from build123d import *

# Parameters (mm, degrees)
SKETCH1_R           = 1.65
BOSS_EXTRUDE1_DEPTH = 16
CUT_EXTRUDE1_START  = -9
CUT_EXTRUDE1_DEPTH  = 9
CUT_EXTRUDE2_DEPTH  = 4
SKETCH4_R           = 1.65
CUT_EXTRUDE3_DEPTH  = 7
CUT_EXTRUDE4_DEPTH  = 4


with BuildPart() as part:
    # Sketch1 → Boss-Extrude1 (new body)
    with BuildSketch(Plane.XY):
        with BuildLine():
            Line((36.52, 7), (33.22, 7))
            ThreePointArc((33.22, 7), (32.866446609, 7.146446609), (32.72, 7.5))
            Line((32.72, 7.5), (32.72, 15.5))
            ThreePointArc((32.72, 15.5), (32.573553391, 15.853553391), (32.22, 16))
            Line((32.22, 16), (4.8, 16))
            ThreePointArc((4.8, 16), (4.446446609, 15.853553391), (4.3, 15.5))
            Line((4.3, 15.5), (4.3, 7.5))
            ThreePointArc((4.3, 7.5), (4.153553391, 7.146446609), (3.8, 7))
            Line((3.8, 7), (0.5, 7))
            ThreePointArc((0.5, 7), (0.146446609, 6.853553391), (0, 6.5))
            Line((0, 6.5), (0, 0.5))
            ThreePointArc((0, 0.5), (0.146446609, 0.146446609), (0.5, 0))
            Line((0.5, 0), (36.52, 0))
            ThreePointArc((36.52, 0), (36.873553391, 0.146446609), (37.02, 0.5))
            Line((37.02, 0.5), (37.02, 6.5))
            ThreePointArc((37.02, 6.5), (36.873553391, 6.853553391), (36.52, 7))
        make_face()
        with Locations((8.81, 11.5)):
            Circle(SKETCH1_R, mode=Mode.SUBTRACT)
        with Locations((28.21, 11.5)):
            Circle(SKETCH1_R, mode=Mode.SUBTRACT)
    extrude(amount=BOSS_EXTRUDE1_DEPTH)

    # Sketch2 → Cut-Extrude1 (cut)
    with BuildSketch(Plane.XY.offset(16).offset(CUT_EXTRUDE1_START)):
        with BuildLine():
            Line((33.22, 7), (3.8, 7))
            ThreePointArc((3.8, 7), (4.153553391, 7.146446609), (4.3, 7.5))
            Line((4.3, 7.5), (4.3, 16))
            Line((4.3, 16), (32.72, 16))
            Line((32.72, 16), (32.72, 7.5))
            ThreePointArc((32.72, 7.5), (32.866446609, 7.146446609), (33.22, 7))
        make_face()
    extrude(amount=CUT_EXTRUDE1_DEPTH, mode=Mode.SUBTRACT)

    # Sketch3 → Cut-Extrude2 (cut)
    with BuildSketch(Plane.XY.offset(7)):
        Polygon((8.6, 8.151368439), (11.5, 9.825684219), (11.5, 13.174315781), (8.6, 14.848631561), (5.7, 13.174315781), (5.7, 9.825684219), align=None)
        Polygon((28, 8.151368439), (30.9, 9.825684219), (30.9, 13.174315781), (28, 14.848631561), (25.1, 13.174315781), (25.1, 9.825684219), align=None)
    extrude(amount=-CUT_EXTRUDE2_DEPTH, mode=Mode.SUBTRACT)

    # Sketch4 → Cut-Extrude3 (cut)
    with BuildSketch(Plane(origin=(0, 7, 0), x_dir=(1, 0, 0), z_dir=(0, 1, 0))):
        with Locations(Location((32.51, -11.5, 0), (0, 0, 270))):
            Circle(SKETCH4_R)
        with Locations(Location((4.51, -11.5, 0), (0, 0, 270))):
            Circle(SKETCH4_R)
    extrude(amount=-CUT_EXTRUDE3_DEPTH, mode=Mode.SUBTRACT)

    # Sketch5 → Cut-Extrude4 (cut)
    with BuildSketch(Plane(origin=(0, 7, 0), x_dir=(1, 0, 0), z_dir=(0, 1, 0))):
        Polygon((32.51, -14.848631561), (35.41, -13.174315781), (35.41, -9.825684219), (32.51, -8.151368439), (29.61, -9.825684219), (29.61, -13.174315781), align=None)
        Polygon((4.51, -14.848631561), (7.41, -13.174315781), (7.41, -9.825684219), (4.51, -8.151368439), (1.61, -9.825684219), (1.61, -13.174315781), align=None)
    extrude(amount=-CUT_EXTRUDE4_DEPTH, mode=Mode.SUBTRACT)


solid = part.part
Build history of the part. All positions in model axes, mm. A direction names the side the tool comes from. Round coordinates to 2 decimals unless told otherwise and drop trailing zeros. Write each loop counter-clockwise with the first axis right and the second up, starting at its lowest first coordinate (ties: lowest second). Pieces come first, ordered by that corner, then holes. Notation, with made-up numbers: M 48.25,73.5 L 105.25,73.5 A8 cw 105.25,83.5 Z; hole C 23,-11.75 d5. An arc over 180 degrees is marked long. Answer as a JSON object with one key per item and string values. Group by question number.
(1) Cut at A-A (y = 11.5). Give the cut face in (x, z), and give its area (3 significant figures).
(2) Drill centre lines: L1, parallel to X at y = 0.8, z = 11.5; L2, parallel to Y at x = 28.21, z = 1.1; L3, parallel to X at y = 12.5, z = 0.75. Where is each one in solid material? Low to high.
(3) Cut at B-B (z = 11.5). Give the cut face in (x, y), and give its area (3 significant figures).
(4) Which spindle directions (+Z, -Z, +X, -X, +Y, -Y) get a long thin tool onto all of the face, cutting with end or side? Do faces 4 (the flat face through (5.7, 12, 5)), 5 (the flat face through (32.72, 11, 3)), 6 (the flat face through (7.41, 5, 12)). Say none if no direction does.
(5) Mould opens along Z. For faces 1 (the flat face through (31.08, 5.028, 8.977)), 2 (the flat face through (18, 8, 0)), 3 (the flat face through (26.57, 14.023, 5.028)) say: pulls with the +Z half, pulls with the -Z half, needs draft (parallel to the pull), parting line crosses it, or undercut.
(6) Cut at D-D (y = 5.25). Give the cut face in (x, z), and give its area (3 significant figures).
(7) Cut at C-C (z = 4.75). Give the cut face in (x, y), and give its area (3 significant figures).
(8) Flat gauge pins, fed straight in: pin 1 (1 mm diameter, centred on y = 11.5, z = 5.5, fed in from +X); pin 2 (4 mm diameter, centred on x = 8.81, y = 11.5, fed in from +Z); pin 3 (6.5 mm diameter, centred on x = 3.5, z = 13, fed in from +Y). Where does each tip first touch, or does it go through?
Responses:
{
 "1": {"outline": "M 4.3,0 L 7.16,0 L 7.16,3 L 5.7,3 L 5.7,7 L 4.3,7 Z; M 10.46,0 L 26.56,0 L 26.56,3 L 25.1,3 L 25.1,7 L 11.5,7 L 11.5,3 L 10.46,3 Z; M 29.86,0 L 32.72,0 L 32.72,7 L 30.9,7 L 30.9,3 L 29.86,3 Z", "area": "133 mm2"},
 "2": {"L1": "x = 0 to 2.86, 6.16 to 30.86, 34.16 to 37.02", "L2": "y = 0 to 9.85, 13.15 to 16", "L3": "x = 4.3 to 7.5, 10.12 to 26.9, 29.52 to 32.72"},
 "3": {"outline": "M 0,0.5 A0.5 ccw 0.5,0 L 2.86,0 L 2.86,3 L 1.61,3 L 1.61,7 L 0.5,7 A0.5 ccw 0,6.5 Z; M 6.16,0 L 30.86,0 L 30.86,3 L 29.61,3 L 29.61,7 L 7.41,7 L 7.41,3 L 6.16,3 Z; M 34.16,0 L 36.52,0 A0.5 ccw 37.02,0.5 L 37.02,6.5 A0.5 ccw 36.52,7 L 35.41,7 L 35.41,3 L 34.16,3 Z", "area": "193 mm2"},
 "4": {"face 4": "+Z", "face 5": "+Z, -Z, +X, +Y", "face 6": "+Y"},
 "5": {"face 1": "undercut", "face 2": "pulls with the -Z half", "face 3": "needs draft"},
 "6": {"outline": "M 0,0 L 37.02,0 L 37.02,16 L 0,16 Z; hole M 1.61,9.83 L 4.51,8.15 L 7.41,9.83 L 7.41,13.17 L 4.51,14.85 L 1.61,13.17 Z; hole M 29.61,9.83 L 32.51,8.15 L 35.41,9.83 L 35.41,13.17 L 32.51,14.85 L 29.61,13.17 Z", "area": "534 mm2"},
 "7": {"outline": "M 0,0.5 A0.5 ccw 0.5,0 L 36.52,0 A0.5 ccw 37.02,0.5 L 37.02,6.5 A0.5 ccw 36.52,7 L 33.22,7 A0.5 cw 32.72,7.5 L 32.72,15.5 A0.5 ccw 32.22,16 L 4.8,16 A0.5 ccw 4.3,15.5 L 4.3,7.5 A0.5 cw 3.8,7 L 0.5,7 A0.5 ccw 0,6.5 Z; hole M 5.7,9.83 L 8.6,8.15 L 11.5,9.83 L 11.5,13.17 L 8.6,14.85 L 5.7,13.17 Z; hole M 25.1,9.83 L 28,8.15 L 30.9,9.83 L 30.9,13.17 L 28,14.85 L 25.1,13.17 Z", "area": "456 mm2"},
 "8": {"pin 1": "stops at x = 32.72", "pin 2": "stops at z = 3", "pin 3": "stops at y = 7"}
}
